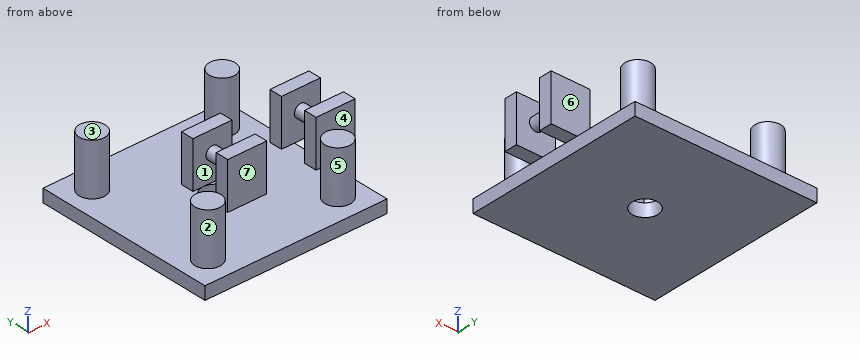
```python
from build123d import *

# Parameters (mm, degrees)
SKETCH1_W           = 70
SKETCH1_H           = 70
SKETCH1_R           = 5
BOSS_EXTRUDE1_DEPTH = 5
SKETCH2_R           = 5
BOSS_EXTRUDE2_DEPTH = 20
CIRPATTERN1_COUNT   = 4
SKETCH3_W           = 15
SKETCH3_H           = 5
BOSS_EXTRUDE3_DEPTH = 18
SKETCH4_R           = 2.5
BOSS_EXTRUDE4_DEPTH = 20


with BuildPart() as part:
    # Sketch1 → Boss-Extrude1 (new body)
    with BuildSketch(Plane.XY):
        Rectangle(SKETCH1_W, SKETCH1_H)
        Circle(SKETCH1_R, mode=Mode.SUBTRACT)
    extrude(amount=BOSS_EXTRUDE1_DEPTH)

    # Sketch2 → Boss-Extrude2 (add)
    with BuildSketch(Plane.XY.offset(5)):
        with Locations((25, 25)):
            Circle(SKETCH2_R)
    boss_extrude2 = extrude(amount=BOSS_EXTRUDE2_DEPTH)

    # CirPattern1: Boss-Extrude2 ×4 about axis
    cirpattern1_axis = Axis((0, 0, 0), (0, 0, 1))
    for i in range(1, CIRPATTERN1_COUNT):
        add(boss_extrude2.rotate(cirpattern1_axis, i * 360 / CIRPATTERN1_COUNT))

    # Sketch3 → Boss-Extrude3 (add)
    with BuildSketch(Plane.XY.offset(5)):
        with Locations((3.5, -7.5)):
            Rectangle(SKETCH3_W, SKETCH3_H)
        with Locations((3.5, 7.5)):
            Rectangle(SKETCH3_W, SKETCH3_H)
        with Locations((37.5, -7.5)):
            Rectangle(SKETCH3_W, SKETCH3_H)
        with Locations((37.5, 7.5)):
            Rectangle(SKETCH3_W, SKETCH3_H)
    extrude(amount=BOSS_EXTRUDE3_DEPTH)

    # Sketch4 → Boss-Extrude4 (add)
    with BuildSketch(Plane(origin=(0, 10, 0), x_dir=(1, 0, 0), z_dir=(0, 1, 0))):
        with Locations(Location((3.5, -15, 0), (0, 0, 270))):
            Circle(SKETCH4_R)
        with Locations(Location((37.5, -15, 0), (0, 0, 270))):
            Circle(SKETCH4_R)
    extrude(amount=-BOSS_EXTRUDE4_DEPTH)


solid = part.part
```
Can you work these out from the model? Positions are in its coordinate system, mm. Face numbers are marked on the shaded views. A direction names the side the tool comes from. Coordinates: 2 decimals unless noted, no trailing zeros. Order: outer loops, then holes, each group sorted by start corner. A loop starts at its lowest first (then second) coordinate and runs counter-clockwise, first axis right, second up. Notation, with made-up numbers: (12, 78) - (31, 78) arc R26 ccw to (31, 115) - close; hole circle Ø4 at (3, 61.25). An arc over 180 degrees is marked (long way). Answer in a Markdown table with one row per item.
1. Suppose I cut it at D-D (z = 21.75). Please give me the cut outline in (x, y), and give its area (3 significant figures).
Reply:
| item | result |
|---|---|
| outline | circle Ø10 at (-25, -25); circle Ø10 at (-25, 25); (-4, -10) - (11, -10) - (11, -5) - (-4, -5) - close; (-4, 5) - (11, 5) - (11, 10) - (-4, 10) - close; circle Ø10 at (25, -25); circle Ø10 at (25, 25); (30, -10) - (45, -10) - (45, -5) - (30, -5) - close; (30, 5) - (45, 5) - (45, 10) - (30, 10) - close |
| area | 614 mm^2 |
2. Suppose I cut it at C-C (x = 37.5). Please give me the cut outline in (y, z), and give its area (3 significant figures).
Reply:
| item | result |
|---|---|
| outline | (-10, 5) - (-5, 5) - (-5, 12.5) - (5, 12.5) - (5, 5) - (10, 5) - (10, 23) - (5, 23) - (5, 17.5) - (-5, 17.5) - (-5, 23) - (-10, 23) - close |
| area | 230 mm^2 |
3. If we mould it in two halves opening along Y, with no side actions, what happens to the marked faces 1, 2, 3 and 4? For each: pulls with the +Y half, pulls with the -Y half, needs draft (parallel to the pull), parting line crosses it, or undercut.
Reply:
| item | result |
|---|---|
| face 1 | undercut |
| face 2 | undercut |
| face 3 | needs draft |
| face 4 | pulls with the -Y half |
4. For pin 1 (3 mm diameter, centred on x = 30, y = -15.5, fed in from -Z); pin 2 (4 mm diameter, centred on x = 37, y = 7, fed in from +Z); pin 3 (4 mm diameter, centred on y = 7, z = 12.5, fed in from -X); pin 4 (4.5 mm diameter, centred on x = 5.5, z = 12.5, fed in from +Y), each with a flat end and sliding along its axis, tell me the tip position at first contact or that it passes through.
Reply:
| item | result |
|---|---|
| pin 1 | stops at z = 0 |
| pin 2 | stops at z = 23 |
| pin 3 | stops at x = -4 |
| pin 4 | stops at y = 10 |
5. Suppose I cut it at B-B (y = 0). Please give me the cut outline in (x, z).
Reply:
| item | result |
|---|---|
| outline | (-35, 0) - (-5, 0) - (-5, 5) - (-35, 5) - close; circle Ø5 at (3.5, 15); (5, 0) - (35, 0) - (35, 5) - (5, 5) - close; circle Ø5 at (37.5, 15) |
6. If I drill on line 1 along X through (y, z) = (0, 2.25); line 2 along X through (y, z) = (-8, 14.5), over which ranges is the centre line in solid material (lowest first)?
Reply:
| item | result |
|---|---|
| line 1 | x = -35 to -5, 5 to 35 |
| line 2 | x = -4 to 11, 30 to 45 |
7. For the marked faces 5, 6 and 7, which set-ups out of +Z, -Z, +X, -X, +Y, -Y let a thin tool reach every point of the face, with its end or its side?
Reply:
| item | result |
|---|---|
| face 5 | +Z |
| face 6 | +Z, +X, -X, +Y |
| face 7 | +Z, +X, -X, -Y |
8. Suppose I cut it at A-A (z = 15). Please give me the cut outline in (x, y), and give its area (3 significant figures).
Reply:
| item | result |
|---|---|
| outline | circle Ø10 at (-25, -25); circle Ø10 at (-25, 25); (-4, -10) - (11, -10) - (11, -5) - (6, -5) - (6, 5) - (11, 5) - (11, 10) - (-4, 10) - (-4, 5) - (1, 5) - (1, -5) - (-4, -5) - close; circle Ø10 at (25, -25); circle Ø10 at (25, 25); (30, -10) - (45, -10) - (45, -5) - (40, -5) - (40, 5) - (45, 5) - (45, 10) - (30, 10) - (30, 5) - (35, 5) - (35, -5) - (30, -5) - close |
| area | 714 mm^2 |
